```python
from build123d import *

# Parameters (mm, degrees)
SKETCH_1_R      = 4
EXTRUDE_1_DEPTH = 16.8
SKETCH_2_W      = 0.8
SKETCH_2_H      = 0.3
EXTRUDE_2_DEPTH = 10


with BuildPart() as part:
    # 草图1 → 凸台-拉伸1 (new body, symmetric)
    with BuildSketch(Plane.XY):
        Circle(SKETCH_1_R)
    extrude(amount=EXTRUDE_1_DEPTH, both=True)

    # 草图2 → 切除-旋转1 (revolve, cut)
    with BuildSketch(Plane(origin=(0, 0, 0), x_dir=(0, 0, -1), z_dir=(1, 0, 0))):
        with Locations((-15.4, 3.85)):
            Rectangle(SKETCH_2_W, SKETCH_2_H)
        with Locations((15.4, 3.85)):
            Rectangle(SKETCH_2_W, SKETCH_2_H)
    revolve(axis=Axis((0, 0, -18.8), (0, 0, 1)), mode=Mode.SUBTRACT)

    # 草图3 → 凸台-拉伸2 (add, symmetric)
    with BuildSketch(Plane(origin=(0, 0, 0), x_dir=(-1, 0, 0), z_dir=(0, 0, 1))):
        with BuildLine():
            Line((5.5, 1.5), (3.708099, 1.5))
            ThreePointArc((3.708099, 1.5), (2.839864, 2.816943), (1.53, 3.695822))
            Line((1.53, 3.695822), (1.53, 5.5))
            Line((1.53, 5.5), (-1.5, 5.5))
            Line((-1.5, 5.5), (-1.5, 3.708099))
            ThreePointArc((-1.5, 3.708099), (-2.839864, -2.816943), (3.695822, -1.53))
            Line((3.695822, -1.53), (5.5, -1.53))
            Line((5.5, -1.53), (5.5, 1.5))
        make_face()
    extrude(amount=EXTRUDE_2_DEPTH, both=True)


solid = part.part
```
Check sheet for the modelled part. Datum: model origin and axes. Units: mm. A direction names the side the tool comes from. Give positions to 0.01 mm unless a question says otherwise; leave off trailing zeros. Order: outer loops, then holes, each group sorted by start corner. A loop starts at its lowest first (then second) coordinate and runs counter-clockwise, first axis right, second up. Notation, with made-up numbers: M 33.25,77.5 L 68.25,77.5 A14 ccw 68.25,103.5 Z; hole C 5,63 d6. An arc over 180 degrees is marked long. Answer in a Markdown table with one row per item.
1) Cross-section at D-D, the plane z = -14. Enter the section's corners in (x, y).
Filled sheet:
| item | result |
|---|---|
| outline | C 0,0 d8 |
2) Release check for a two-part mould opening along Z. For faces 1 (the cylindrical face through (3.612, -0.802, 15.394)), 2 (the cylindrical face through (3.815, 1.201, 16.307)), 3 (the flat face through (0, -5, 10)) record: +Z half, -Z half, draft (parallel to the pull), parting line (faces both ways), or undercut.
Filled sheet:
| item | result |
|---|---|
| face 1 | undercut |
| face 2 | draft |
| face 3 | +Z half |
3) Access from +Z, -Z, +X, -X, +Y, -Y to the whole of each face (thin tool, end or side, straight path). Record for faces 4 (the flat face through (-5, 1.53, 0)), 5 (the cylindrical face through (3.815, 1.201, -16.293)), 6 (the cylindrical face through (3.612, -0.802, -15.406)), 7 (the flat face through (-5, -1.5, 0)).
Filled sheet:
| item | result |
|---|---|
| face 4 | +Z, -Z, -X, +Y |
| face 5 | -Z |
| face 6 | none |
| face 7 | +Z, -Z, -X, -Y |
4) Gauge pin test, flat ends, axial feed: P1, Ø0.5, axis at x = -5, z = 4, coming from the +Y side; P2, Ø0.9, axis at x = -0.5, y = -4.5, coming from the +Z side; P3, Ø0.9, axis at x = -4.5, y = 0.5, coming from the -Z side. Record the tip position at first contact, or that the pin passes through.
Filled sheet:
| item | result |
|---|---|
| P1 | stops at y = 1.53 |
| P2 | stops at z = 10 |
| P3 | stops at z = -10 |
5) Cross-section at B-B, the plane z = 9. Enter the section's corners in (x, y).
Filled sheet:
| item | result |
|---|---|
| outline | M -5.5,-1.5 L -3.71,-1.5 A4 ccw -1.53,-3.7 L -1.53,-5.5 L 1.5,-5.5 L 1.5,-3.71 A4 ccw long -3.7,1.53 L -5.5,1.53 Z |
6) Cross-section at A-A, the plane y = 0. Enter the section's corners in (x, z).
Filled sheet:
| item | result |
|---|---|
| outline | M -5.5,-10 L -4,-10 L -4,-15 L -3.7,-15 L -3.7,-15.8 L -4,-15.8 L -4,-16.8 L 4,-16.8 L 4,-15.8 L 3.7,-15.8 L 3.7,-15 L 4,-15 L 4,15 L 3.7,15 L 3.7,15.8 L 4,15.8 L 4,16.8 L -4,16.8 L -4,15.8 L -3.7,15.8 L -3.7,15 L -4,15 L -4,10 L -5.5,10 Z |
7) Thickness scan on L1, parallel to X at y = -4.5, z = 5.5; L2, parallel to Y at x = -4.5, z = 3; L3, parallel to X at y = -1.5, z = -12.5. Record the ranges inside material, lowest first. Write a range as [from, to].
Filled sheet:
| item | result |
|---|---|
| L1 | x = [-1.53, 1.5] |
| L2 | y = [-1.5, 1.53] |
| L3 | x = [-3.71, 3.71] |
